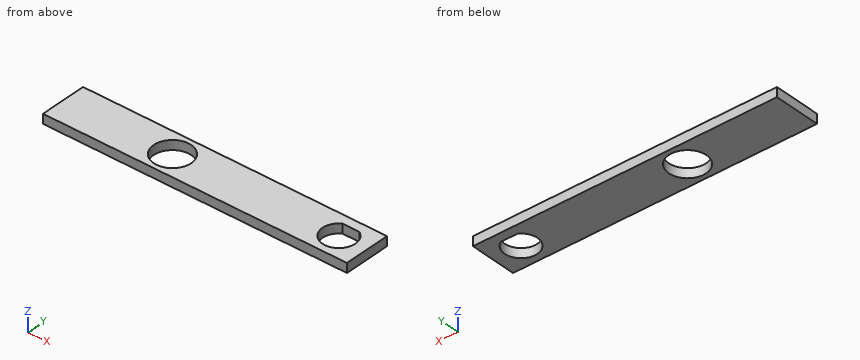
from build123d import *

# Parameters (mm, degrees)
SKETCH1_W           = 65
SKETCH1_H           = 10
SKETCH1_R           = 4
BOSS_EXTRUDE2_DEPTH = 2


with BuildPart() as part:
    # Sketch1 → Boss-Extrude2 (new body)
    with BuildSketch(Plane.XY):
        with Locations((9.1, 0)):
            Rectangle(SKETCH1_W, SKETCH1_H)
        Circle(SKETCH1_R, mode=Mode.SUBTRACT)
        with BuildLine():
            Line((33.797224362, 3), (37.402775638, 3))
            ThreePointArc((37.402775638, 3), (35.6, -3.5), (33.797224362, 3))
        make_face(mode=Mode.SUBTRACT)
    extrude(amount=BOSS_EXTRUDE2_DEPTH)


solid = part.part
Work out the finished part from the listing and answer in its coordinate system (mm). Give positions to 0.01 mm unless a question says otherwise; leave off trailing zeros. Loops run counter-clockwise (first coordinate to the right, second up) from the corner with the lowest first, then second, coordinate; pieces in that order, holes last. Notation, with made-up numbers: (48, 56.25) -> (84, 56.25) arc R16 ccw to (84, 74.25) -> close; hole circle Ø1 at (68, -4). An arc over 180 degrees is marked (long way). Use a Markdown table: item, result. Add a question column.
1) The part is cut by section D-D, the plane x = 0. Determine the outline of the cut face in (y, z), plus the area to 3 significant figures.
2) Consider line 1 along X through (y, z) = (1.25, 0.9); line 2 along X through (y, z) = (-2.5, 0.55); line 3 along Y through (x, z) = (0, 1.25). Determine where each line is inside the solid, lowest interval first.
3) The part is cut by section B-B, the plane y = 0. Determine the outline of the cut face in (x, z).
4) This flat-tipped pin is pushed along its axis until it touches: P1, Ø5, axis at x = 0, y = 0, coming from the -Z side. Where does it stop, or does it pass through?
5) The part is cut by section C-C, the plane z = 1. Determine the outline of the cut face in (x, y).
6) The part is cut by section A-A, the plane x = 35.6. Determine the outline of the cut face in (y, z), plus the area to 3 significant figures.
Reported:
| question | item | result |
|---|---|---|
| 1 | outline | (-5, 0) -> (-4, 0) -> (-4, 2) -> (-5, 2) -> close; (4, 0) -> (5, 0) -> (5, 2) -> (4, 2) -> close |
| 1 | area | 4.00 mm^2 |
| 2 | line 1 | x = -23.4 to -3.8, 3.8 to 32.33, 38.87 to 41.6 |
| 2 | line 2 | x = -23.4 to -3.12, 3.12 to 33.15, 38.05 to 41.6 |
| 2 | line 3 | y = -5 to -4, 4 to 5 |
| 3 | outline | (-23.4, 0) -> (-4, 0) -> (-4, 2) -> (-23.4, 2) -> close; (4, 0) -> (32.1, 0) -> (32.1, 2) -> (4, 2) -> close; (39.1, 0) -> (41.6, 0) -> (41.6, 2) -> (39.1, 2) -> close |
| 4 | P1 | passes through |
| 5 | outline | (-23.4, -5) -> (41.6, -5) -> (41.6, 5) -> (-23.4, 5) -> close; hole circle Ø8 at (0, 0); hole (33.8, 3) arc R3.5 ccw (long way) to (37.4, 3) -> close |
| 6 | outline | (-5, 0) -> (-3.5, 0) -> (-3.5, 2) -> (-5, 2) -> close; (3, 0) -> (5, 0) -> (5, 2) -> (3, 2) -> close |
| 6 | area | 7.00 mm^2 |
